For this review, take the finished solid that the model builds, in its own axes (mm). Face numbers are marked on the shaded views. A direction names the side the tool comes from. Give positions to 0.01 mm unless a question says otherwise; leave off trailing zeros. Write each loop counter-clockwise with the first axis right and the second up, starting at its lowest first coordinate (ties: lowest second). Pieces come first, ordered by that corner, then holes. Notation, with made-up numbers: M 43.25,55.5 L 48.25,55.5 A13 ccw 48.25,69.5 Z; hole C 51,46.25 d11. An arc over 180 degrees is marked long. Use one line per item in the form item = value. Start each with the question number.
Q1. Tool access review of the marked faces 4 and 5: name each direction out of +Z, -Z, +X, -X, +Y, -Y from which nothing blocks a thin tool from reaching the whole face with its end or side.
Q2. Consider section C-C on z = 19. Write out the cut boundary in (x, y), and give its area (3 significant figures).
Q3. Clearance check with flat-ended pins moving along their axes: pin 1 Ø1.5 at (x, z) = (9.5, -17) entering from -Y (3 decimals); pin 2 Ø6 at (x, z) = (18, -14.5) entering from -Y; pin 3 Ø2 at (x, z) = (6.5, 13.5) entering from -Y. State where each tip first meets the part, or that it passes through.
Q4. Consider section A-A on y = 16.5. Write out the cut boundary in (x, z).
Q5. For probe 1 along Z at (x, y) = (9.75, 0.5); probe 2 along Z at (x, y) = (14.75, 10.5); probe 3 along Y at (x, z) = (15.5, 3.5), list the stretches that pass through material, from the lowest coordinate up. Write a range as [from, to].
Q6. Consider section B-B on z = -1.5. Write out the cut boundary in (x, y), and give its area (3 significant figures).
Q7. Mouldability with a two-part tool opening along Y and no side actions: class the marked faces 1, 2 and 3 as released by +Y, released by -Y, zero draft, split by the parting line, or undercut.
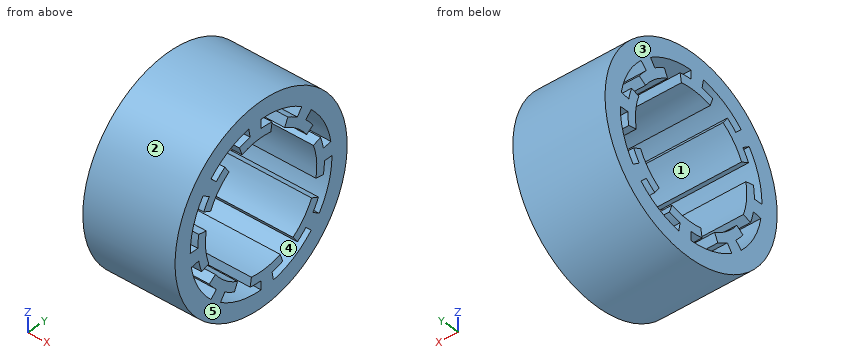
```python
from build123d import *

# Parameters (mm, degrees)
SKETCH1_R           = 21.59
SKETCH1_R_2         = 17.78
BOSS_EXTRUDE1_DEPTH = 20.32
BOSS_EXTRUDE2_DEPTH = 20.32
CIRPATTERN1_COUNT   = 8


with BuildPart() as part:
    # Sketch1 → Boss-Extrude1 (new body)
    with BuildSketch(Plane.YZ):
        with Locations(Location((0, 0, 0), (0, 0, 270))):
            Circle(SKETCH1_R)
        with Locations(Location((0, 0, 0), (0, 0, 270))):
            Circle(SKETCH1_R_2, mode=Mode.SUBTRACT)
    extrude(amount=BOSS_EXTRUDE1_DEPTH)

    # Sketch3 → Boss-Extrude2 (add)
    with BuildSketch(Plane.YZ):
        with BuildLine():
            Line((-3.087464599, 17.509881849), (-2.75666482, 15.633823079))
            ThreePointArc((-2.75666482, 15.633823079), (-4.108752341, 15.334072492), (-5.429569775, 14.917620355))
            Line((-5.429569775, 14.917620355), (-4.778021402, 13.127505912))
            ThreePointArc((-4.778021402, 13.127505912), (-1.217565726, 13.916839932), (2.425865042, 13.75776431))
            Line((2.425865042, 13.75776431), (2.75666482, 15.633823079))
            ThreePointArc((2.75666482, 15.633823079), (1.383597416, 15.814590832), (0, 15.875))
            Line((0, 15.875), (0, 17.78))
            ThreePointArc((0, 17.78), (-1.549629106, 17.712341732), (-3.087464599, 17.509881849))
        make_face()
    boss_extrude2 = extrude(amount=BOSS_EXTRUDE2_DEPTH)

    # CirPattern1: Boss-Extrude2 ×8 about axis
    cirpattern1_axis = Axis((0, 0, 0), (1, 0, 0))
    for i in range(1, CIRPATTERN1_COUNT):
        add(boss_extrude2.rotate(cirpattern1_axis, i * 360 / CIRPATTERN1_COUNT))


solid = part.part
```
Working result:
q1.face_4 = +X, -X
q1.face_5 = +Z, -Z, +X, +Y, -Y
q2.outline = M 0,-10.25 L 20.32,-10.25 L 20.32,10.25 L 0,10.25 Z
q2.area = 417 mm²
q3.pin_1 = -14.215
q3.pin_2 = -18.27
q3.pin_3 = -17.6
q4.outline = M 0,-13.92 L 20.32,-13.92 L 20.32,-6.62 L 0,-6.62 Z; M 0,0 L 20.32,0 L 20.32,2.91 L 0,2.91 Z; M 0,6.62 L 20.32,6.62 L 20.32,13.92 L 0,13.92 Z
q5.probe_1 = [-21.58, -13.96], [13.96, 15.87], [17.77, 21.58]
q5.probe_2 = [-18.86, -14.35], [-11.91, -9.21], [9.21, 18.86]
q5.probe_3 = [-21.3, -17.43], [13.52, 15.48], [17.43, 21.3]
q6.outline = M 0,-21.54 L 20.32,-21.54 L 20.32,-13.89 L 0,-13.89 Z; M 0,13.89 L 20.32,13.89 L 20.32,15.8 L 0,15.8 Z; M 0,17.72 L 20.32,17.72 L 20.32,21.54 L 0,21.54 Z
q6.area = 272 mm²
q7.face_1 = undercut
q7.face_2 = split by the parting line
q7.face_3 = zero draft
